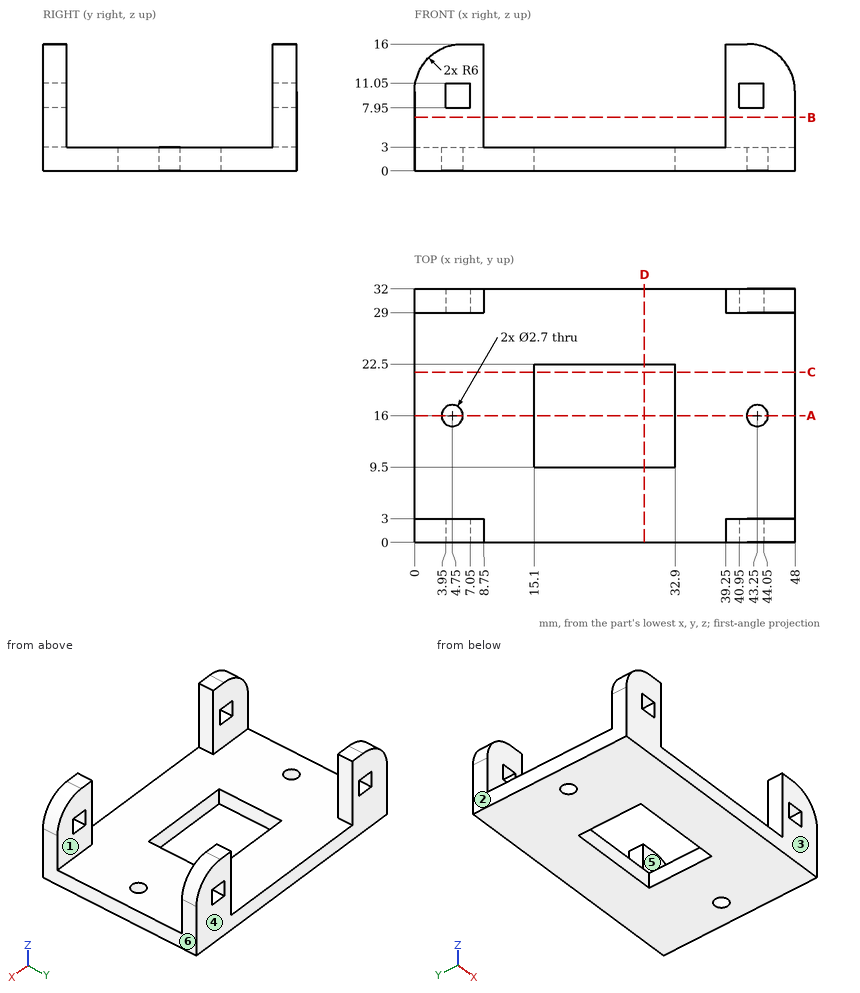
Geometry check sheet. Reference: drawing and pictorial views, mm from the part's lowest x, y, z. A direction names the side the tool comes from. Give positions to 0.01 mm unless a question says otherwise; leave off trailing zeros. Write each loop counter-clockwise with the first axis right and the second up, starting at its lowest first coordinate (ties: lowest second). Pieces come first, ordered by that corner, then holes. Notation, with made-up numbers: M 18.5,27 L 66.5,27 A8 ccw 66.5,41 Z; hole C 59,47 d9. An arc over 180 degrees is marked long. Put each result on its own line as item: value. Start each with the question number.
1. Section check B-B (z = 6.75). Record the cut outline in (x, y).
2. Draft check along Y on the marked faces 1, 2, 3 and 4. Enter one of: +Y half, -Y half, draft (parallel to the pull), parting line (faces both ways), or undercut.
3. Scan lines: line 1 along Y through (x, z) = (41.5, 12.75); line 2 along Y through (x, z) = (4.75, 2.15); line 3 along Z through (x, y) = (12, 12). Record each from-to range of solid material in increasing order. Write a range as [from, to].
4. Set-up check for the marked faces 5 and 6: record each of +Z, -Z, +X, -X, +Y, -Y from which the full face is reachable in a straight line by a thin tool's end or side.
5. Section check A-A (y = 16). Record the cut outline in (x, z).
6. Go/stop test with a flat-tipped pin: pin 1 Ø16 at (x, y) = (15, 15) entering from +Z. Record where the tip stops, or that it passes through.
7. Section check C-C (y = 21.5). Record the cut outline in (x, z).
8. Section check D-D (x = 29). Record the cut outline in (y, z), and give its area (3 significant figures).
Answer list:
1. outline: M 0,0 L 8.75,0 L 8.75,3 L 0,3 Z; M 0,29 L 8.75,29 L 8.75,32 L 0,32 Z; M 39.25,0 L 48,0 L 48,3 L 39.25,3 Z; M 39.25,29 L 48,29 L 48,32 L 39.25,32 Z
2. face 1: undercut
2. face 2: draft
2. face 3: -Y half
2. face 4: +Y half
3. line 1: [0, 3], [29, 32]
3. line 2: [0, 14.65], [17.35, 32]
3. line 3: [0, 3]
4. face 5: +Z, +X, -X
4. face 6: +Z, -Z, +X, +Y, -Y
5. outline: M 0,0 L 3.4,0 L 3.4,3 L 0,3 Z; M 6.1,0 L 15.1,0 L 15.1,3 L 6.1,3 Z; M 32.9,0 L 41.9,0 L 41.9,3 L 32.9,3 Z; M 44.6,0 L 48,0 L 48,3 L 44.6,3 Z
6. pin 1: z = 3
7. outline: M 0,0 L 15.1,0 L 15.1,3 L 0,3 Z; M 32.9,0 L 48,0 L 48,3 L 32.9,3 Z
8. outline: M 0,0 L 9.5,0 L 9.5,3 L 0,3 Z; M 22.5,0 L 32,0 L 32,3 L 22.5,3 Z
8. area: 57.0 mm2
